from build123d import *

# Parameters (mm, degrees)
SKETCH1_W           = 70.5
SKETCH1_H           = 81
BOSS_EXTRUDE1_DEPTH = 3
SKETCH2_W           = 5
SKETCH2_H           = 3
BOSS_EXTRUDE2_DEPTH = 5
SKETCH3_W           = 5
SKETCH3_H           = 3
BOSS_EXTRUDE3_DEPTH = 5
BOSS_EXTRUDE4_DEPTH = 3


with BuildPart() as part:
    # Sketch1 → Boss-Extrude1 (new body)
    with BuildSketch(Plane(origin=(0, 0, 0), x_dir=(1, 0, 0), z_dir=(0, 1, 0))):
        with Locations((35.25, -40.5)):
            Rectangle(SKETCH1_W, SKETCH1_H)
    extrude(amount=BOSS_EXTRUDE1_DEPTH)

    # Sketch2 → Boss-Extrude2 (add)
    with BuildSketch(Plane.XY.offset(81)):
        with Locations((5.54, 1.5)):
            Rectangle(SKETCH2_W, SKETCH2_H)
        with Locations((64.96, 1.5)):
            Rectangle(SKETCH2_W, SKETCH2_H)
    extrude(amount=BOSS_EXTRUDE2_DEPTH)

    # Sketch3 → Boss-Extrude3 (add)
    with BuildSketch(Plane(origin=(0, 0, 0), x_dir=(-1, 0, 0), z_dir=(0, 0, -1))):
        with Locations((-5.54, 1.5)):
            Rectangle(SKETCH3_W, SKETCH3_H)
        with Locations((-64.96, 1.5)):
            Rectangle(SKETCH3_W, SKETCH3_H)
    extrude(amount=BOSS_EXTRUDE3_DEPTH)

    # Sketch4 → Boss-Extrude4 (add)
    with BuildSketch(Plane(origin=(0, 3, 0), x_dir=(1, 0, 0), z_dir=(0, 1, 0))):
        Polygon((0, 0), (0, 5), (-5, 5), (-5, -86), (0, -86), (0, -81), align=None)
        Polygon((70.5, 5), (70.5, 0), (70.5, -81), (70.5, -86), (75.5, -86), (75.5, 0), (75.5, 5), align=None)
    extrude(amount=-BOSS_EXTRUDE4_DEPTH)


solid = part.part
Source: CAD feature listing. Evaluate the final solid. Frame: model axes, mm. A direction names the side the tool comes from. Round coordinates to 2 decimals unless told otherwise and drop trailing zeros. Loops run counter-clockwise (first coordinate to the right, second up) from the corner with the lowest first, then second, coordinate; pieces in that order, holes last.
Q1. Mould query, pull axis X, two halves, no side actions, for faces 4 (the face through (35, 0, 40)), 5 (the face through (67.46, 1, -2)), 6 (the face through (-5, 2, 40)). Classes: pulls with the +X half, pulls with the -X half, needs draft (parallel to the pull), parting line crosses it, or undercut.
Q2. Ray query, line 1 (Z direction, x = 18, y = 0.45). Return the intervals inside material, ascending.
Q3. Access query for faces 1 (the face through (62.46, 1, 83)), 2 (the face through (6, 2, 86)), 3 (the face through (1, 1, 0)). Directions: +Z, -Z, +X, -X, +Y, -Y. A direction counts if a zero-diameter tool reaches every point of the face in a straight line with its end or side. Return the directions, or none.
Q4. Section A-A, the plane y = 0.65. Return loops of the section in (x, z).
Q5. Section B-B, the plane x = 42. Return loops of the section in (y, z), plus the area to 3 significant figures.
Q6. First-contact query: P1, Ø1.5, axis at x = 38.5, y = 1.5, coming from the +Z side. Flat tip, straight axial feed; report the tip coordinate or a pass-through.
Solutions:
1. face 4: needs draft
1. face 5: undercut
1. face 6: pulls with the -X half
2. line 1: z = 0 to 81
3. face 1: +Z, +Y, -Y
3. face 2: +Z, +X, -X, +Y, -Y
3. face 3: -Z, +Y, -Y
4. outline: (-5, -5) - (0, -5) - (0, 0) - (3.04, 0) - (3.04, -5) - (8.04, -5) - (8.04, 0) - (62.46, 0) - (62.46, -5) - (67.46, -5) - (67.46, 0) - (70.5, 0) - (70.5, -5) - (75.5, -5) - (75.5, 86) - (70.5, 86) - (70.5, 81) - (67.46, 81) - (67.46, 86) - (62.46, 86) - (62.46, 81) - (8.04, 81) - (8.04, 86) - (3.04, 86) - (3.04, 81) - (0, 81) - (0, 86) - (-5, 86) - close
5. outline: (0, 0) - (3, 0) - (3, 81) - (0, 81) - close
5. area: 243 mm2
6. P1: stops at z = 81
